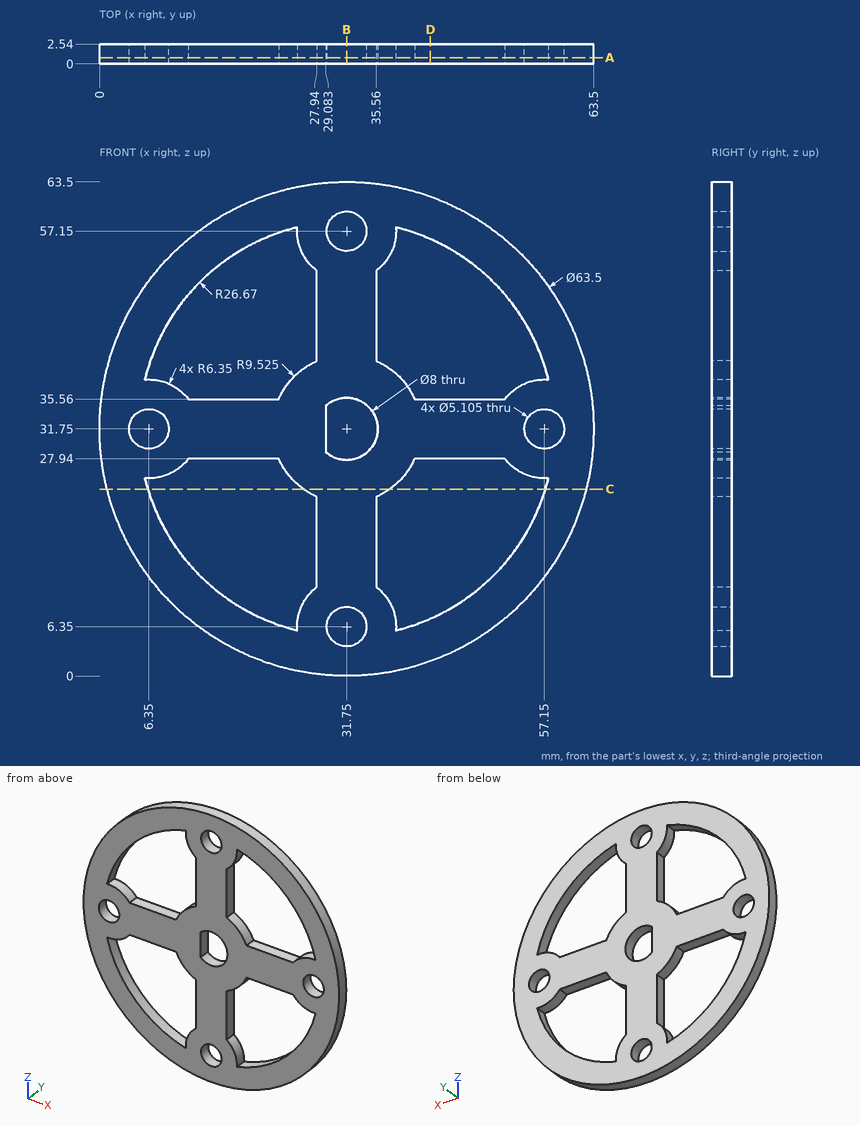
Here's the drawing with two shaded views (mm, measured from the low corner). I have some questions. Coordinates: 2 decimals unless noted, no trailing zeros. Loops run counter-clockwise (first coordinate to the right, second up) from the corner with the lowest first, then second, coordinate; pieces in that order, holes last. Notation, with made-up numbers: (-35.5, 87) - (22.5, 87) arc R20 cw to (22.5, 113) - close; hole circle Ø2 at (37.5, 74). An arc over 180 degrees is marked (long way). Answer as CSV lines item,"result". Start each with the question number.
1) For pin 1 (1.5 mm diameter, centred on y = 1.5, z = 48.5, fed in from -X); pin 2 (1.3 mm diameter, centred on x = 15.5, y = 1.5, fed in from +Z); pin 3 (0.8 mm diameter, centred on y = 2, z = 44, fed in from -X) (1 decimal); pin 4 (6 mm diameter, centred on x = 31.75, z = 6.35, fed in from -Y), each with a flat end and sliding along its axis, tell me the tip position at first contact or that it passes through.
2) Suppose I cut it at B-B (x = 31.75). Please give me the cut outline in (y, z).
3) Suppose I cut it at D-D (x = 42.5). Please give me the cut outline in (y, z) (1 decimal).
4) I need wall thicknesses on line 1 (X direction, y = 0.8, z = 31.75); line 2 (Z direction, x = 31.75, y = 1.75); line 3 (Z direction, x = 50.5, y = 0.9) (1 decimal). Which ranges of each line are inside material? Lowest first, please. Write a range as from..to.
5) Suppose I cut it at A-A (y = 0.8). Count the separate pieces of the cut face and the enclosed holes in it, plus the area to 3 significant figures.
6) Suppose I cut it at C-C (z = 24). Please give me the cut outline in (x, y).
Check result:
1,pin 1,"stops at x = 4.33"
1,pin 2,"stops at z = 59.4"
1,pin 3,"stops at x = 2.3"
1,pin 4,"stops at y = 0"
2,outline,"(0, 0) - (2.54, 0) - (2.54, 3.8) - (0, 3.8) - close; (0, 8.9) - (2.54, 8.9) - (2.54, 27.75) - (0, 27.75) - close; (0, 35.75) - (2.54, 35.75) - (2.54, 54.6) - (0, 54.6) - close; (0, 59.7) - (2.54, 59.7) - (2.54, 63.5) - (0, 63.5) - close"
3,outline,"(0, 1.9) - (2.5, 1.9) - (2.5, 7.3) - (0, 7.3) - close; (0, 27.9) - (2.5, 27.9) - (2.5, 35.6) - (0, 35.6) - close; (0, 56.2) - (2.5, 56.2) - (2.5, 61.6) - (0, 61.6) - close"
4,line 1,"x = 0..3.8, 8.9..29.08, 35.75..54.6, 59.7..63.5"
4,line 2,"z = 0..3.8, 8.9..27.75, 35.75..54.6, 59.7..63.5"
4,line 3,"z = 6.1..12.8, 27.9..35.6, 50.7..57.4"
5,separate pieces,"1"
5,enclosed holes,"9"
5,area,"1,710 mm²"
6,outline,"(0.96, 0) - (6.23, 0) - (6.23, 2.54) - (0.96, 2.54) - close; (26.21, 0) - (37.29, 0) - (37.29, 2.54) - (26.21, 2.54) - close; (57.27, 0) - (62.54, 0) - (62.54, 2.54) - (57.27, 2.54) - close"
